Autodesk Inventor part; units mm, degrees
ref_plane "YZ Plane" through (0, 0, 0) normal (1, 0, 0) x (0, 1, 0)
ref_plane "XZ Plane" through (0, 0, 0) normal (0, 1, 0) x (-1, 0, 0)
ref_plane "XY Plane" through (0, 0, 0) normal (0, 0, 1) x (1, 0, 0)
sketch "Sketch1" plane through (0, 0, 0) normal (0, 0, 1) x (1, 0, 0)
  line L0 (-65.5, -40.5) -> (65.5, -40.5)
  line L1 (65.5, -40.5) -> (65.5, 40.5)
  line L2 (65.5, 40.5) -> (-65.5, 40.5)
  line L3 (-65.5, 40.5) -> (-65.5, -40.5)
  line L4 (-65.5, -40.5) -> (65.5, 40.5) construction
  line L5 (65.5, -40.5) -> (-65.5, 40.5) construction
  point P0 (0, 0)
  dimension "d0" = 131
  dimension "d1" = 81
extrude "Extrusion1" add sketch "Sketch1" along normal blind 3
sketch "Sketch2" plane through (0, 0, 3) normal (0, 0, 1) x (1, 0, 0)
  line L0 (65.5, -40.5) -> (65.5, 40.5)
  line L1 (65.5, 40.5) -> (65.5, 24.3)
  line L2 (65.5, 24.3) -> (68.5, 24.3)
  line L3 (68.5, 24.3) -> (68.5, 40.5)
  line L4 (68.5, 40.5) -> (65.5, 40.5)
  line L5 (65.5, 8.1) -> (65.5, -8.1)
  line L6 (65.5, -8.1) -> (68.5, -8.1)
  line L7 (68.5, -8.1) -> (68.5, 8.1)
  line L8 (68.5, 8.1) -> (65.5, 8.1)
  line L9 (65.5, -24.3) -> (65.5, -40.5)
  line L10 (65.5, -40.5) -> (68.5, -40.5)
  line L11 (68.5, -40.5) -> (68.5, -24.3)
  line L12 (68.5, -24.3) -> (65.5, -24.3)
  line L13 (0, -60.9) -> (0, 60.9)
  line L14 (-91.7, 0) -> (91.7, 0)
  line L15 (-65.5, -40.5) -> (-65.5, 40.5)
  line L16 (-65.5, 40.5) -> (-65.5, 24.3)
  line L17 (-65.5, 24.3) -> (-68.5, 24.3)
  line L18 (-68.5, 24.3) -> (-68.5, 40.5)
  line L19 (-68.5, 40.5) -> (-65.5, 40.5)
  line L20 (-65.5, 8.1) -> (-65.5, -8.1)
  line L21 (-65.5, -8.1) -> (-68.5, -8.1)
  line L22 (-68.5, -8.1) -> (-68.5, 8.1)
  line L23 (-68.5, 8.1) -> (-65.5, 8.1)
  line L24 (-65.5, -24.3) -> (-65.5, -40.5)
  line L25 (-65.5, -40.5) -> (-68.5, -40.5)
  line L26 (-68.5, -40.5) -> (-68.5, -24.3)
  line L27 (-68.5, -24.3) -> (-65.5, -24.3)
  line L28 (65.5, 40.5) -> (-65.5, 40.5)
  line L29 (65.5, 40.5) -> (50.9444, 40.5)
  line L30 (50.9444, 40.5) -> (50.9444, 43.5)
  line L31 (50.9444, 43.5) -> (65.5, 43.5)
  line L32 (65.5, 43.5) -> (65.5, 40.5)
  line L33 (36.3889, 40.5) -> (21.8333, 40.5)
  line L34 (21.8333, 40.5) -> (21.8333, 43.5)
  line L35 (21.8333, 43.5) -> (36.3889, 43.5)
  line L36 (36.3889, 43.5) -> (36.3889, 40.5)
  line L37 (7.2778, 40.5) -> (-7.2778, 40.5)
  line L38 (-7.2778, 40.5) -> (-7.2778, 43.5)
  line L39 (-7.2778, 43.5) -> (7.2778, 43.5)
  line L40 (7.2778, 43.5) -> (7.2778, 40.5)
  line L41 (-21.8333, 40.5) -> (-36.3889, 40.5)
  line L42 (-36.3889, 40.5) -> (-36.3889, 43.5)
  line L43 (-36.3889, 43.5) -> (-21.8333, 43.5)
  line L44 (-21.8333, 43.5) -> (-21.8333, 40.5)
  line L45 (-50.9444, 40.5) -> (-65.5, 40.5)
  line L46 (-65.5, 40.5) -> (-65.5, 43.5)
  line L47 (-65.5, 43.5) -> (-50.9444, 43.5)
  line L48 (-50.9444, 43.5) -> (-50.9444, 40.5)
  line L49 (-68.5, -40.5) -> (-65.5, -40.5)
  line L50 (65.5, -40.5) -> (-65.5, -40.5)
  line L51 (65.5, -40.5) -> (50.9444, -40.5)
  line L52 (50.9444, -40.5) -> (50.9444, -43.5)
  line L53 (50.9444, -43.5) -> (65.5, -43.5)
  line L54 (65.5, -43.5) -> (65.5, -40.5)
  line L55 (36.3889, -40.5) -> (21.8333, -40.5)
  line L56 (36.3889, -43.5) -> (36.3889, -40.5)
  line L57 (21.8333, -43.5) -> (36.3889, -43.5)
  line L58 (21.8333, -40.5) -> (21.8333, -43.5)
  line L59 (7.2778, -40.5) -> (-7.2778, -40.5)
  line L60 (7.2778, -43.5) -> (7.2778, -40.5)
  line L61 (-7.2778, -43.5) -> (7.2778, -43.5)
  line L62 (-7.2778, -40.5) -> (-7.2778, -43.5)
  line L63 (-21.8333, -40.5) -> (-36.3889, -40.5)
  line L64 (-21.8333, -43.5) -> (-21.8333, -40.5)
  line L65 (-36.3889, -43.5) -> (-21.8333, -43.5)
  line L66 (-36.3889, -40.5) -> (-36.3889, -43.5)
  line L67 (-50.9444, -40.5) -> (-65.5, -40.5)
  line L68 (-50.9444, -43.5) -> (-50.9444, -40.5)
  line L69 (-65.5, -43.5) -> (-50.9444, -43.5)
  line L70 (-65.5, -40.5) -> (-65.5, -43.5)
  point P0 (0, 0)
  point P1 (65.5, 0)
  point P2 (65.5, -32.4)
  point P3 (65.5, 0)
  point P4 (-65.5, 0)
  point P5 (-65.5, -32.4)
  point P6 (-65.5, 0)
  point P7 (0, 43.5)
  point P8 (0, 40.5)
  point P9 (0, -43.5)
  point P10 (0, -40.5)
  point P11 (-21.8333, -40.5)
  point P12 (7.2778, -40.5)
  point P13 (-7.2778, -40.5)
  point P14 (-7.2778, 40.5)
  point P15 (7.2778, 40.5)
  point P16 (-65.5, 8.1)
  point P17 (-21.8333, 40.5)
  dimension "d4" = 3
  dimension "d5" = 16.2
  dimension "d6" = 3
  dimension "d7" = 16.2
  dimension "d10" = 3
  dimension "d11" = 16.2
  dimension "d14" = 3
  dimension "d15" = 14.5556
  dimension "d16" = 3
  dimension "d17" = 14.5556
  dimension "d21" = 3
  dimension "d22" = 14.5556
  dimension "d26" = 3
  dimension "d27" = 14.5556
  dimension "d31" = 3
  dimension "d32" = 14.5556
  dimension "d36" = 14.5556
  dimension "d37" = 14.5556
extrude "Extrusion2" add sketch "Sketch2" against normal up to surface (3 mm away) contours L0 L12 L11 L10 | L54 L53 L52 L50 | L0 L14 L7 L6 | L56 L57 L58 L50 | L0 L8 L7 L14 | L60 L61 L13 L50 | L0 L4 L3 L2 | L13 L61 L62 L50 | L28 L38 L39 L13 | L13 L39 L40 L28 | L15 L21 L22 L14 | L14 L22 L23 L15 | L28 L30 L31 L32 | L64 L65 L66 L50 | L34 L35 L36 L28 | L28 L42 L43 L44 | L15 L25 L26 L27 | L17 L18 L19 L15 | L50 L68 L69 L70 | L46 L47 L48 L28
equation "\"d4\" = d2"
equation "\"d5\" = 0.2 * d1"
equation "\"d6\" = d8"
equation "\"d7\" = 0.2 * d9"
equation "\"d10\" = d12"
equation "\"d11\" = 0.2 * d13"
equation "\"d14\" = d4"
equation "\"d15\" = 0.111111 * d0"
equation "\"d16\" = d18"
equation "\"d17\" = d15"
equation "\"d21\" = d23"
equation "\"d22\" = d15"
equation "\"d26\" = d28"
equation "\"d27\" = d15"
equation "\"d31\" = d33"
equation "\"d32\" = d15"
equation "\"d36\" = d15"
equation "\"d37\" = d15"
equation "\"d8\" = d2"
equation "\"d9\" = d1"
equation "\"d12\" = d2"
equation "\"d13\" = d1"
equation "\"d18\" = d20"
equation "\"d20\" = d2"
equation "\"d23\" = d25"
equation "\"d25\" = d2"
equation "\"d28\" = d30"
equation "\"d30\" = d2"
equation "\"d33\" = d35"
equation "\"d35\" = d2"
properties part number "bottom"
Could you check a few things on this model? Use its own coordinates, in mm. A direction names the side the tool comes from. Give positions to 0.01 mm unless a question says otherwise; leave off trailing zeros. Order: outer loops, then holes, each group sorted by start corner. A loop starts at its lowest first (then second) coordinate and runs counter-clockwise, first axis right, second up.
Q1. I'm going to push flat-ended pins straight in: P1, Ø0.9, axis at y = 42, z = 1.5, coming from the -X side; P2, Ø0.9, axis at x = 47, z = 1, coming from the -Y side; P3, Ø0.9, axis at x = 66.5, z = 1.5, coming from the +Y side. Where does each tip first touch, or does it pass through?
Q2. Suppose I cut it at B-B, the plane x = -38.5. Write out the boundary of the cut face in (y, z).
Q3. Suppose I cut it at A-A, the plane y = -22.5. Write out the boundary of the cut face in (x, z), and give its area (3 significant figures).
Q4. For faces 1 (the flat face through (-67, 8.1, 2)), 2 (the flat face through (21.833, 42, 2)), 3 (the flat face through (-21.833, -42, 2)), 4 (the flat face through (67, -40.5, 2)), 5 (the flat face through (-67, 40.5, 2)), which set-ups out of +Z, -Z, +X, -X, +Y, -Y let a thin tool reach every point of the face, with its end or its side?
Q5. If I drill on line 1 along Y through (x, z) = (40, 2); line 2 along X through (y, z) = (-20, 1.6), over which ranges is the centre line in solid material (lowest first)?
Q6. We'd pull the mould along X, two halves only. Please class faces 6 (the flat face through (15, 40.5, 1)), 7 (the flat face through (65.5, 16, 1)), 8 (the flat face through (-21.833, 42, 2)), 9 (the flat face through (-67, -24.3, 2)): +X half, -X half, draft (parallel to the pull), parting line (faces both ways), or undercut.
Solution:
1. P1: stops at x = -65.5
1. P2: stops at y = -40.5
1. P3: stops at y = 40.5
2. outline: (-40.5, 0) - (40.5, 0) - (40.5, 3) - (-40.5, 3) - close
3. outline: (-65.5, 0) - (65.5, 0) - (65.5, 3) - (-65.5, 3) - close
3. area: 393 mm2
4. face 1: +Z, -Z, -X
4. face 2: +Z, -Z, +Y
4. face 3: +Z, -Z, -Y
4. face 4: +Z, -Z, +X, -Y
4. face 5: +Z, -Z, -X, +Y
5. line 1: y = -40.5 to 40.5
5. line 2: x = -65.5 to 65.5
6. face 6: undercut
6. face 7: +X half
6. face 8: undercut
6. face 9: draft
